The model under review builds one solid part; all positions refer to its coordinate system, in mm. Round coordinates to 2 decimals unless told otherwise and drop trailing zeros. Write each loop counter-clockwise with the first axis right and the second up, starting at its lowest first coordinate (ties: lowest second). Pieces come first, ordered by that corner, then holes. Notation, with made-up numbers: M 42,-6.75 L 75,-6.75 A16 cw 75,17.25 Z; hole C 66,57 d6. An arc over 180 degrees is marked long. Write item = value, one per line. Start each with the question number.
Item 1: To check wall thickness, follow line 1 along Y through (x, z) = (0.2, 0.45); line 2 along X through (y, z) = (0.8, 0.3). State the ranges of each line that lie inside material, in increasing order.
Item 2: Take a section at B-B, the plane y = 0.8. Give the boundary of the cut face in (x, z).
Item 3: Take a section at A-A, the plane x = 0.2. Give the boundary of the cut face in (y, z), plus the area to 3 significant figures.
Item 4: The part is to be moulded in two halves that separate along X. For faces 1 (the flat face through (0, 0, 0.035)), 2 (the cylindrical face through (0.772, 0.98, 0.331)), say which applies: +X half, -X half, draft (parallel to the pull), parting line (faces both ways), or undercut.
from build123d import *

# Parameters (mm, degrees)
PAD_DEPTH                        = 0.6
SKETCH001_R                      = 0.6
POCKET_DEPTH                     = 0.601
SKETCH002_R                      = 0.2848
POCKET001_DEPTH                  = 45.871741
SKETCH002_LINEARPATTERN_2_R      = 0.2848
POCKET001_LINEARPATTERN_2_DEPTH  = 45.871741
SKETCH002_LINEARPATTERN_3_R      = 0.2848
POCKET001_LINEARPATTERN_3_DEPTH  = 45.871741
SKETCH002_LINEARPATTERN_4_R      = 0.2848
POCKET001_LINEARPATTERN_4_DEPTH  = 45.871741
SKETCH002_LINEARPATTERN_5_R      = 0.2848
POCKET001_LINEARPATTERN_5_DEPTH  = 45.871741
SKETCH002_LINEARPATTERN_6_R      = 0.2848
POCKET001_LINEARPATTERN_6_DEPTH  = 45.871741
SKETCH002_LINEARPATTERN_7_R      = 0.2848
POCKET001_LINEARPATTERN_7_DEPTH  = 45.871741
SKETCH002_LINEARPATTERN_8_R      = 0.2848
POCKET001_LINEARPATTERN_8_DEPTH  = 45.871741
SKETCH002_LINEARPATTERN_9_R      = 0.2848
POCKET001_LINEARPATTERN_9_DEPTH  = 45.871741
SKETCH002_LINEARPATTERN_10_R     = 0.2848
POCKET001_LINEARPATTERN_10_DEPTH = 45.871741


with BuildPart() as part:
    # Sketch → Pad (new body)
    with BuildSketch(Plane.XY):
        Polygon((-8, -8), (8, -8), (8, 8), (-7.6, 8), (-8, 7.6), align=None)
    extrude(amount=PAD_DEPTH)

    # Sketch001 → Pocket (cut, through all)
    with BuildSketch(Plane.XY):
        with Locations((0.2, 0.8)):
            Circle(SKETCH001_R)
    extrude(amount=POCKET_DEPTH, mode=Mode.SUBTRACT)

    # Sketch002 → Pocket001 (cut, through all)
    with BuildSketch(Plane.XY):
        with Locations((-8, 6.75)):
            Circle(SKETCH002_R)
    pocket001 = extrude(amount=POCKET001_DEPTH, mode=Mode.SUBTRACT)

    # Sketch002 LinearPattern 2 → Pocket001 LinearPattern 2 (cut, through all)
    with BuildSketch(Plane(origin=(0, -1.5, 0), x_dir=(1, 0, 0), z_dir=(0, 0, 1))):
        with Locations((-8, 6.75)):
            Circle(SKETCH002_LINEARPATTERN_2_R)
    pocket001_linearpattern_2 = extrude(amount=POCKET001_LINEARPATTERN_2_DEPTH, mode=Mode.SUBTRACT)

    # Sketch002 LinearPattern 3 → Pocket001 LinearPattern 3 (cut, through all)
    with BuildSketch(Plane(origin=(0, -3, 0), x_dir=(1, 0, 0), z_dir=(0, 0, 1))):
        with Locations((-8, 6.75)):
            Circle(SKETCH002_LINEARPATTERN_3_R)
    pocket001_linearpattern_3 = extrude(amount=POCKET001_LINEARPATTERN_3_DEPTH, mode=Mode.SUBTRACT)

    # Sketch002 LinearPattern 4 → Pocket001 LinearPattern 4 (cut, through all)
    with BuildSketch(Plane(origin=(0, -4.5, 0), x_dir=(1, 0, 0), z_dir=(0, 0, 1))):
        with Locations((-8, 6.75)):
            Circle(SKETCH002_LINEARPATTERN_4_R)
    pocket001_linearpattern_4 = extrude(amount=POCKET001_LINEARPATTERN_4_DEPTH, mode=Mode.SUBTRACT)

    # Sketch002 LinearPattern 5 → Pocket001 LinearPattern 5 (cut, through all)
    with BuildSketch(Plane(origin=(0, -6, 0), x_dir=(1, 0, 0), z_dir=(0, 0, 1))):
        with Locations((-8, 6.75)):
            Circle(SKETCH002_LINEARPATTERN_5_R)
    pocket001_linearpattern_5 = extrude(amount=POCKET001_LINEARPATTERN_5_DEPTH, mode=Mode.SUBTRACT)

    # Sketch002 LinearPattern 6 → Pocket001 LinearPattern 6 (cut, through all)
    with BuildSketch(Plane(origin=(0, -7.5, 0), x_dir=(1, 0, 0), z_dir=(0, 0, 1))):
        with Locations((-8, 6.75)):
            Circle(SKETCH002_LINEARPATTERN_6_R)
    pocket001_linearpattern_6 = extrude(amount=POCKET001_LINEARPATTERN_6_DEPTH, mode=Mode.SUBTRACT)

    # Sketch002 LinearPattern 7 → Pocket001 LinearPattern 7 (cut, through all)
    with BuildSketch(Plane(origin=(0, -9, 0), x_dir=(1, 0, 0), z_dir=(0, 0, 1))):
        with Locations((-8, 6.75)):
            Circle(SKETCH002_LINEARPATTERN_7_R)
    pocket001_linearpattern_7 = extrude(amount=POCKET001_LINEARPATTERN_7_DEPTH, mode=Mode.SUBTRACT)

    # Sketch002 LinearPattern 8 → Pocket001 LinearPattern 8 (cut, through all)
    with BuildSketch(Plane(origin=(0, -10.5, 0), x_dir=(1, 0, 0), z_dir=(0, 0, 1))):
        with Locations((-8, 6.75)):
            Circle(SKETCH002_LINEARPATTERN_8_R)
    pocket001_linearpattern_8 = extrude(amount=POCKET001_LINEARPATTERN_8_DEPTH, mode=Mode.SUBTRACT)

    # Sketch002 LinearPattern 9 → Pocket001 LinearPattern 9 (cut, through all)
    with BuildSketch(Plane(origin=(0, -12, 0), x_dir=(1, 0, 0), z_dir=(0, 0, 1))):
        with Locations((-8, 6.75)):
            Circle(SKETCH002_LINEARPATTERN_9_R)
    pocket001_linearpattern_9 = extrude(amount=POCKET001_LINEARPATTERN_9_DEPTH, mode=Mode.SUBTRACT)

    # Sketch002 LinearPattern 10 → Pocket001 LinearPattern 10 (cut, through all)
    with BuildSketch(Plane(origin=(0, -13.5, 0), x_dir=(1, 0, 0), z_dir=(0, 0, 1))):
        with Locations((-8, 6.75)):
            Circle(SKETCH002_LINEARPATTERN_10_R)
    pocket001_linearpattern_10 = extrude(amount=POCKET001_LINEARPATTERN_10_DEPTH, mode=Mode.SUBTRACT)

    # Mirrored: Pocket001, Pocket001 LinearPattern 2, Pocket001 LinearPattern 3, Pocket001 LinearPattern 4, Pocket001 LinearPattern 5, Pocket001 LinearPattern 6, Pocket001 LinearPattern 7, Pocket001 LinearPattern 8, Pocket001 LinearPattern 9, Pocket001 LinearPattern 10 across Sketch002 V_Axis
    add(pocket001.mirror(Plane(origin=(0, 0, 0), x_dir=(0, 0, 1), z_dir=(1, 0, 0))), mode=Mode.SUBTRACT)
    add(pocket001_linearpattern_2.mirror(Plane(origin=(0, 0, 0), x_dir=(0, 0, 1), z_dir=(1, 0, 0))), mode=Mode.SUBTRACT)
    add(pocket001_linearpattern_3.mirror(Plane(origin=(0, 0, 0), x_dir=(0, 0, 1), z_dir=(1, 0, 0))), mode=Mode.SUBTRACT)
    add(pocket001_linearpattern_4.mirror(Plane(origin=(0, 0, 0), x_dir=(0, 0, 1), z_dir=(1, 0, 0))), mode=Mode.SUBTRACT)
    add(pocket001_linearpattern_5.mirror(Plane(origin=(0, 0, 0), x_dir=(0, 0, 1), z_dir=(1, 0, 0))), mode=Mode.SUBTRACT)
    add(pocket001_linearpattern_6.mirror(Plane(origin=(0, 0, 0), x_dir=(0, 0, 1), z_dir=(1, 0, 0))), mode=Mode.SUBTRACT)
    add(pocket001_linearpattern_7.mirror(Plane(origin=(0, 0, 0), x_dir=(0, 0, 1), z_dir=(1, 0, 0))), mode=Mode.SUBTRACT)
    add(pocket001_linearpattern_8.mirror(Plane(origin=(0, 0, 0), x_dir=(0, 0, 1), z_dir=(1, 0, 0))), mode=Mode.SUBTRACT)
    add(pocket001_linearpattern_9.mirror(Plane(origin=(0, 0, 0), x_dir=(0, 0, 1), z_dir=(1, 0, 0))), mode=Mode.SUBTRACT)
    add(pocket001_linearpattern_10.mirror(Plane(origin=(0, 0, 0), x_dir=(0, 0, 1), z_dir=(1, 0, 0))), mode=Mode.SUBTRACT)


with BuildPart() as part_1:
    # Body placement: moved
    add(part.part.moved(Location((0, 0, 0.0348))))


solid = part_1.part
Response values:
q1.line_1 = -8 to 0.2, 1.4 to 8
q1.line_2 = -7.72 to -0.4, 0.8 to 7.72
q2.outline = M -7.72,0.03 L -0.4,0.03 L -0.4,0.63 L -7.72,0.63 Z; M 0.8,0.03 L 7.72,0.03 L 7.72,0.63 L 0.8,0.63 Z
q3.outline = M -8,0.03 L 0.2,0.03 L 0.2,0.63 L -8,0.63 Z; M 1.4,0.03 L 8,0.03 L 8,0.63 L 1.4,0.63 Z
q3.area = 8.88 mm2
q4.face_1 = draft
q4.face_2 = undercut
